Work out the finished part from the listing and answer in its coordinate system (mm). A direction names the side the tool comes from. Round coordinates to 2 decimals unless told otherwise and drop trailing zeros. Write each loop counter-clockwise with the first axis right and the second up, starting at its lowest first coordinate (ties: lowest second). Pieces come first, ordered by that corner, then holes.
1. Flat-ended cylindrical pins translate along their axes: pin 1 Ø1.4 at (y, z) = (3, 19.5) entering from +X; pin 2 Ø8 at (y, z) = (42, -1) entering from +X; pin 3 Ø6 at (y, z) = (44.5, 2.5) entering from -X. Find the tip coordinate at first contact, or state that the pin passes through.
2. A tool of negligible diameter and unlimited length cuts with its end or side. For faces 4 (the face through (-3, 15.6, 6)), 5 (the face through (0, 5, 21.513)), 6 (the face through (9.258, 5, 19)), 7 (the face through (-0.5, 44, 0)), 8 (the face through (0, 0, 0)), from which of +Z, -Z, +X, -X, +Y, -Y can it reach the whole face along a straight path? Write none if from no direction.
3. Determine the mould class of faces 1 (the face through (0, 9.5, 14)), 2 (the face through (-9.258, 5, 19)), 3 (the face through (-3.83, 25.95, -5)) for opening direction Z: pulls with the +Z half, pulls with the -Z half, needs draft (parallel to the pull), parting line crosses it, or undercut.
4. Find section A-A (y = 22.5). Write down the section's boundary in (x, z).
5. Straight lines are drawn through the part: probe 1 along Y at (x, z) = (-6.25, 13); probe 2 along Y at (x, z) = (-4, 7); probe 3 along Z at (x, y) = (4, 7). For each, find the intervals that lie inside material, in ascending order.
```python
from build123d import *

# Parameters (mm, degrees)
SKETCH1_R           = 12.8
BOSS_EXTRUDE1_DEPTH = 9.5
BOSS_EXTRUDE2_DEPTH = 1.8
SKETCH3_R           = 12.75
BOSS_EXTRUDE3_DEPTH = 4.3
SKETCH4_R           = 6.3
BOSS_EXTRUDE4_DEPTH = 22
CHAMFER1_SIZE       = 1
CHAMFER2_SIZE       = 0.5
SKETCH5_W           = 18.515372874
SKETCH5_H           = 4.830097271
BOSS_EXTRUDE5_DEPTH = 10
SKETCH6_W           = 1
SKETCH6_H           = 10
BOSS_EXTRUDE6_DEPTH = 12
CHAMFER3_SIZE       = 4


with BuildPart() as part:
    # Sketch1 → Boss-Extrude1 (new body)
    with BuildSketch(Plane(origin=(0, 0, 0), x_dir=(1, 0, 0), z_dir=(0, 1, 0))):
        with Locations(Location((0, 0, 0), (0, 0, 270))):
            Circle(SKETCH1_R)
    extrude(amount=BOSS_EXTRUDE1_DEPTH)

    # Sketch2 → Boss-Extrude2 (add)
    with BuildSketch(Plane(origin=(0, 9.5, 0), x_dir=(1, 0, 0), z_dir=(0, 1, 0))):
        with BuildLine():
            Line((12.8, -23.8), (-12.8, -23.8))
            Line((-12.8, -23.8), (-12.8, 0))
            ThreePointArc((-12.8, 0), (0, 12.8), (12.8, 0))
            Line((12.8, 0), (12.8, -23.8))
        make_face()
    extrude(amount=BOSS_EXTRUDE2_DEPTH)

    # Sketch3 → Boss-Extrude3 (add)
    with BuildSketch(Plane(origin=(0, 11.3, 0), x_dir=(1, 0, 0), z_dir=(0, 1, 0))):
        with Locations(Location((0, 0, 0), (0, 0, 90))):
            Circle(SKETCH3_R)
    extrude(amount=BOSS_EXTRUDE3_DEPTH)

    # Sketch4 → Boss-Extrude4 (add)
    with BuildSketch(Plane(origin=(0, 15.6, 0), x_dir=(1, 0, 0), z_dir=(0, 1, 0))):
        with Locations(Location((0, 0, 0), (0, 0, 270))):
            Circle(SKETCH4_R)
    extrude(amount=BOSS_EXTRUDE4_DEPTH)

    # Chamfer1
    chamfer1_edges = [part.edges().sort_by_distance(p)[0] for p in [
        (0, 37.6, -6.3),
    ]]
    chamfer(chamfer1_edges, length=CHAMFER1_SIZE)

    # Chamfer2
    chamfer2_edges = [part.edges().sort_by_distance(p)[0] for p in [
        (0, 0, -12.8),
        (0, 15.6, 12.75),
    ]]
    chamfer(chamfer2_edges, length=CHAMFER2_SIZE)

    # Sketch5 → Boss-Extrude5 (add)
    with BuildSketch(Plane.XZ.offset(-9.5)):
        with Locations((0, 19.097773841)):
            Rectangle(SKETCH5_W, SKETCH5_H)
    extrude(amount=BOSS_EXTRUDE5_DEPTH)

    # Sketch6 → Boss-Extrude6 (add)
    with BuildSketch(Plane(origin=(0, 37.6, 0), x_dir=(1, 0, 0), z_dir=(0, 1, 0))):
        Rectangle(SKETCH6_W, SKETCH6_H)
    extrude(amount=BOSS_EXTRUDE6_DEPTH)

    # Chamfer3
    chamfer3_edges = [part.edges().sort_by_distance(p)[0] for p in [
        (-12.8, 10.4, 23.8),
        (12.8, 10.4, 23.8),
    ]]
    chamfer(chamfer3_edges, length=CHAMFER3_SIZE)


solid = part.part
```
Worked answers:
1. pin 1: stops at x = 9.26
1. pin 2: stops at x = 0.5
1. pin 3: stops at x = -0.5
2. face 4: +Y
2. face 5: +Z, +X, -X, -Y
2. face 6: +Z, +X, -Y
2. face 7: +Z, -Z, -X, +Y
2. face 8: -Z, +X, -X, -Y
3. face 1: undercut
3. face 2: needs draft
3. face 3: parting line crosses it
4. outline: circle Ø12.6 at (0, 0)
5. probe 1: y = 9.5 to 11.3
5. probe 2: y = 0 to 15.6
5. probe 3: z = -12.16 to 12.16, 16.68 to 21.51
